The listing builds one solid part. Answer for the finished solid, in the listing's coordinates (mm). Face numbers are marked on the shaded views. A direction names the side the tool comes from. Round coordinates to 2 decimals unless told otherwise and drop trailing zeros. Order: outer loops, then holes, each group sorted by start corner. A loop starts at its lowest first (then second) coordinate and runs counter-clockwise, first axis right, second up. Notation, with made-up numbers: M 32.5,46.5 L 87.5,46.5 A24 cw 87.5,67.5 Z; hole C 19.5,26 d7. An arc over 180 degrees is marked long. Put each result on its own line as item: value. Start each with the question number.
1. The part is cut by section C-C (x = -12). Give the vertices of the cut face in (y, z).
2. The part is cut by section D-D (z = -8.5). Give the vertices of the cut face in (x, y).
3. The part is cut by section B-B (z = 7.5). Give the vertices of the cut face in (x, y).
4. The part is cut by section A-A (y = -14). Give the vertices of the cut face in (x, z), then the cut area to 3 significant figures.
5. Which of the six approach directions +Z, -Z, +X, -X, +Y, -Y give full straight-line access (tool end or side, diameter ignored) to the marked faces 5, 6 and 7?
6. Consider line 1 (X direction, y = -11, z = 8); line 2 (Y direction, x = -0.75, z = -12.5); line 3 (Z direction, x = -12.5, y = -15.5). Determine where each line is inside the solid, lowest interval first.
7. Each of these flat-tipped pins is pushed along its axis until it touches: pin 1 Ø10 at (y, z) = (-17.5, -2.5) entering from -X; pin 2 Ø1.5 at (y, z) = (-9, -11) entering from +X; pin 3 Ø12 at (x, z) = (6.5, 0.5) entering from +Y; pin 4 Ø1 at (x, z) = (0.5, 10) entering from -Y. Where does it stop, or does it pass through?
8. The mould has two halves that part along X. Classify the marked faces 1, 2, 3 and 4: +X half, -X half, draft (parallel to the pull), parting line (faces both ways), or undercut.
from build123d import *

# Parameters (mm, degrees)
ESQUISSE1_W                = 30
ESQUISSE1_H                = 6
BOSS_EXTRU_1_DEPTH         = 17.5
ESQUISSE3_R                = 1.8
BOSS_EXTRU_2_DEPTH         = 5
R_P_TITION_LIN_AIRE1_COUNT = 2
R_P_TITION_LIN_AIRE1_PITCH = 23


with BuildPart() as part:
    # Esquisse1 → Boss.-Extru.1 (new, symmetric)
    with BuildSketch(Plane.XY):
        with Locations((0, -3)):
            Rectangle(ESQUISSE1_W, ESQUISSE1_H)
    extrude(amount=BOSS_EXTRU_1_DEPTH, both=True)

    # Esquisse3 → Boss.-Extru.2 (add)
    with BuildSketch(Plane(origin=(14, 0, 0), x_dir=(0, 0, -1), z_dir=(1, 0, 0))):
        with BuildLine():
            Line((-17.5, -6), (17.5, -6))
            Line((17.5, -6), (-3.901517868, -24.817916067))
            ThreePointArc((-3.901517868, -24.817916067), (-8.286202576, -25.856849364), (-11.600005345, -22.803399907))
            Line((-11.600005345, -22.803399907), (-17.5, -6))
        make_face()
        with Locations((-7.071067812, -21.213203436)):
            Circle(ESQUISSE3_R, mode=Mode.SUBTRACT)
    boss_extru_2 = extrude(amount=-BOSS_EXTRU_2_DEPTH)

    # Répétition linéaire1: Boss.-Extru.2 ×2
    with Locations(*[(-i * R_P_TITION_LIN_AIRE1_PITCH, 0, 0) for i in range(1, R_P_TITION_LIN_AIRE1_COUNT)]):
        add(boss_extru_2)


solid = part.part
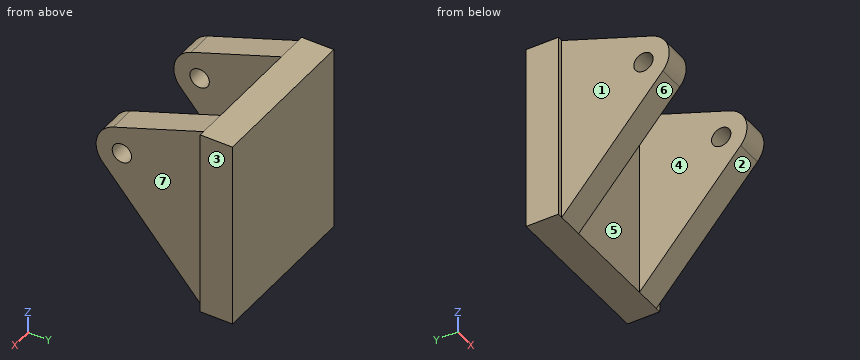
Resolved:
1. outline: M -24.82,3.9 L -6,-17.5 L 0,-17.5 L 0,17.5 L -6,17.5 L -22.8,11.6 A4.8 ccw Z; hole C -21.21,7.07 d3.6
2. outline: M -15,-6 L -14,-6 L -14,-13.91 L -9,-13.91 L -9,-6 L 9,-6 L 9,-13.91 L 14,-13.91 L 14,-6 L 15,-6 L 15,0 L -15,0 Z
3. outline: M -15,-6 L -14,-6 L -14,-19.47 L -9,-19.47 L -9,-6 L 9,-6 L 9,-19.47 L 14,-19.47 L 14,-6 L 15,-6 L 15,0 L -15,0 Z; M -14,-25.99 L -9,-25.99 L -9,-22.96 L -14,-22.96 Z; M 9,-25.99 L 14,-25.99 L 14,-22.96 L 9,-22.96 Z
4. outline: M -14,-8.4 L -9,-8.4 L -9,14.69 L -14,14.69 Z; M 9,-8.4 L 14,-8.4 L 14,14.69 L 9,14.69 Z
4. area: 231 mm2
5. face 5: +Z, -Z, -Y
5. face 6: -Z, +X, -X, -Y
5. face 7: +Z, -Z, +X, -Y
6. line 1: -14 to -9, 9 to 14
6. line 2: -6 to 0
6. line 3: -6.7 to 14.16
7. pin 1: x = -14
7. pin 2: x = 14
7. pin 3: y = 0
7. pin 4: y = -6
8. face 1: -X half
8. face 2: draft
8. face 3: +X half
8. face 4: undercut
